```python
from build123d import *

# Parameters (mm, degrees)
ESQUISSE3_W              = 78
ESQUISSE3_H              = 56
BOSS_EXTRU_2_DEPTH       = 45
ESQUISSE4_R              = 34
ENL_V_MAT_EXTRU_1_DEPTH  = 30
ESQUISSE5_W              = 35.5
ESQUISSE5_H              = 35.5
ENL_V_MAT_EXTRU_2_DEPTH  = 15
ENL_V_MAT_EXTRU_5_DEPTH  = 10
ESQUISSE12_W             = 68
ESQUISSE12_H             = 18
ENL_V_MAT_EXTRU_6_DEPTH  = 30
ESQUISSE13_R             = 1.671466639
ENL_V_MAT_EXTRU_7_DEPTH  = 62.75
ESQUISSE15_R             = 1.5
ENL_V_MAT_EXTRU_8_DEPTH  = 62.75
ESQUISSE16_W             = 8
ESQUISSE16_H             = 8
ENL_V_MAT_EXTRU_9_DEPTH  = 4
ESQUISSE17_R             = 1.5
ENL_V_MAT_EXTRU_10_DEPTH = 41.5
ESQUISSE18_R             = 1.5
ENL_V_MAT_EXTRU_11_DEPTH = 41.5
ESQUISSE19_W             = 8
ESQUISSE19_H             = 8
ENL_V_MAT_EXTRU_12_DEPTH = 4
ENL_V_MAT_EXTRU_13_DEPTH = 46


with BuildPart() as part:
    # Esquisse3 → Boss.-Extru.2 (new body)
    with BuildSketch(Plane.XY):
        Rectangle(ESQUISSE3_W, ESQUISSE3_H)
    extrude(amount=BOSS_EXTRU_2_DEPTH)

    # Esquisse4 → Enlèv. mat.-Extru.1 (cut)
    with BuildSketch(Plane.XY.offset(45)):
        with Locations((0, -10)):
            Circle(ESQUISSE4_R)
    extrude(amount=-ENL_V_MAT_EXTRU_1_DEPTH, mode=Mode.SUBTRACT)

    # Esquisse5 → Enlèv. mat.-Extru.2 (cut)
    with BuildSketch(Plane(origin=(0, 0, 0), x_dir=(-1, 0, 0), z_dir=(0, 0, -1))):
        with Locations((0, -10.25)):
            Rectangle(ESQUISSE5_W, ESQUISSE5_H)
    extrude(amount=-ENL_V_MAT_EXTRU_2_DEPTH, mode=Mode.SUBTRACT)

    # Esquisse8 → Enlèv. mat.-Extru.5 (cut)
    with BuildSketch(Plane(origin=(0, 0, 0), x_dir=(-1, 0, 0), z_dir=(0, 0, -1))):
        Polygon((-22.75, -28), (-22.75, 12.5), (22.75, 12.5), (22.75, -28), (39, -28), (39, 28), (-39, 28), (-39, -28), align=None)
    extrude(amount=-ENL_V_MAT_EXTRU_5_DEPTH, mode=Mode.SUBTRACT)

    # Esquisse12 → Enlèv. mat.-Extru.6 (cut)
    with BuildSketch(Plane.XY.offset(45)):
        with Locations((0, -19)):
            Rectangle(ESQUISSE12_W, ESQUISSE12_H)
    extrude(amount=-ENL_V_MAT_EXTRU_6_DEPTH, mode=Mode.SUBTRACT)

    # Esquisse13 → Enlèv. mat.-Extru.7 (cut, through all)
    with BuildSketch(Plane.ZY.offset(22.75)):
        with Locations((5, -23)):
            Circle(ESQUISSE13_R)
    extrude(amount=-ENL_V_MAT_EXTRU_7_DEPTH, mode=Mode.SUBTRACT)

    # Esquisse15 → Enlèv. mat.-Extru.8 (cut, through all)
    with BuildSketch(Plane.ZY.offset(22.75)):
        with Locations((5, 2.5)):
            Circle(ESQUISSE15_R)
    extrude(amount=-ENL_V_MAT_EXTRU_8_DEPTH, mode=Mode.SUBTRACT)

    # Esquisse16 → Enlèv. mat.-Extru.9 (cut)
    with BuildSketch(Plane.XY.offset(15)):
        with Locations((-17.75, 7.5)):
            Rectangle(ESQUISSE16_W, ESQUISSE16_H)
    extrude(amount=-ENL_V_MAT_EXTRU_9_DEPTH, mode=Mode.SUBTRACT)

    # Esquisse17 → Enlèv. mat.-Extru.10 (cut, through all)
    with BuildSketch(Plane(origin=(0, 12.5, 0), x_dir=(1, 0, 0), z_dir=(0, 1, 0))):
        with Locations((-12.75, -5)):
            Circle(ESQUISSE17_R)
    extrude(amount=-ENL_V_MAT_EXTRU_10_DEPTH, mode=Mode.SUBTRACT)

    # Esquisse18 → Enlèv. mat.-Extru.11 (cut, through all)
    with BuildSketch(Plane(origin=(0, 12.5, 0), x_dir=(1, 0, 0), z_dir=(0, 1, 0))):
        with Locations((12.75, -5)):
            Circle(ESQUISSE18_R)
    extrude(amount=-ENL_V_MAT_EXTRU_11_DEPTH, mode=Mode.SUBTRACT)

    # Esquisse19 → Enlèv. mat.-Extru.12 (cut)
    with BuildSketch(Plane.XY.offset(15)):
        with Locations((17.75, 7.5)):
            Rectangle(ESQUISSE19_W, ESQUISSE19_H)
    extrude(amount=-ENL_V_MAT_EXTRU_12_DEPTH, mode=Mode.SUBTRACT)

    # Esquisse20 → Enlèv. mat.-Extru.13 (cut, through all)
    with BuildSketch(Plane.XY.offset(45)):
        Polygon((-39, 3), (-39, 28), (-14, 28), align=None)
    enl_v_mat_extru_13 = extrude(amount=-ENL_V_MAT_EXTRU_13_DEPTH, mode=Mode.SUBTRACT)

    # Symétrie1: Enlèv. mat.-Extru.13 across plane
    add(enl_v_mat_extru_13.mirror(Plane(origin=(0, 0, 0), x_dir=(0, 0, 1), z_dir=(1, 0, 0))), mode=Mode.SUBTRACT)


solid = part.part
```
Could you check a few things on this model? Use its own coordinates, in mm. A direction names the side the tool comes from. Give positions to 0.01 mm unless a question says otherwise; leave off trailing zeros. Order: outer loops, then holes, each group sorted by start corner. A loop starts at its lowest first (then second) coordinate and runs counter-clockwise, first axis right, second up.
Q1. I'm going to push flat-ended pins straight in: P1, Ø5, axis at x = -3.5, z = 6, coming from the +Y side; P2, Ø4.5, axis at y = 8, z = 13.5, coming from the +X side; P3, Ø10, axis at y = 12.5, z = 18, coming from the +X side; P4, Ø6, axis at x = -3.5, y = 6.5, coming from the -Z side. Where does each tip first touch, or does it pass through?
Q2. Suppose I cut it at D-D, the plane z = 12.5. Write out the boundary of the cut face in (x, y).
Q3. For faces 1 (the cylindrical face through (0.75, 23.99, 30.21)), 2 (the flat face through (0, 12.5, 5)), 3 (the flat face through (22.75, -8, 5)), which set-ups out of +Z, -Z, +X, -X, +Y, -Y let a thin tool reach every point of the face, with its end or its side?
Q4. If I drill on line 1 along X through (y, z) = (9.6, 5); line 2 along Y through (x, z) = (-20, 5); line 3 along Z through (x, y) = (-12.75, 10.5), over which ranges is the centre line in solid material (lowest first)?
Q5. Suppose I cut it at A-A, the plane y = -18. Write out the boundary of the cut face in (x, z).
Q6. Suppose I cut it at C-C, the plane x = -30. Write out the boundary of the cut face in (y, z).
Q7. Suppose I cut it at B-B, the plane z = 5. Count the separate pieces of the cut face and the enclosed holes in it, and give its area (3 significant figures).
Q8. We'd pull the mould along Y, two halves only. Please class faces 4 (the flat face through (19, 8, 11)), 5 (the flat face through (35, -28, 21)), 6 (the flat face through (-9, 23, 45)): +Y half, -Y half, draft (parallel to the pull), parting line (faces both ways), or undercut.
Solution:
1. P1: stops at y = 12.5
1. P2: stops at x = 36.25
1. P3: stops at x = 34.5
1. P4: stops at z = 0
2. outline: (-39, -28) - (-17.75, -28) - (-17.75, 3.5) - (-21.75, 3.5) - (-21.75, 11.5) - (-13.75, 11.5) - (-13.75, 7.5) - (13.75, 7.5) - (13.75, 11.5) - (21.75, 11.5) - (21.75, 3.5) - (17.75, 3.5) - (17.75, -28) - (39, -28) - (39, 3) - (14, 28) - (-14, 28) - (-39, 3) - close
3. face 1: +Z, -Y
3. face 2: -Z, +X, -X, +Y
3. face 3: -Z, +X, +Y, -Y
4. line 1: x = -22.75 to -14.25, -11.25 to 11.25, 14.25 to 22.75
4. line 2: y = -28 to -24.67, -21.33 to 1, 4 to 12.5
4. line 3: z = 0 to 3.5, 6.5 to 15
5. outline: (-39, 10) - (-22.75, 10) - (-22.75, 0) - (-17.75, 0) - (-17.75, 15) - (-34, 15) - (-34, 45) - (-39, 45) - close; (17.75, 0) - (22.75, 0) - (22.75, 10) - (39, 10) - (39, 45) - (34, 45) - (34, 15) - (17.75, 15) - close
6. outline: (-28, 10) - (12, 10) - (12, 45) - (6, 45) - (6, 15) - (-28, 15) - close
7. separate pieces: 7
7. enclosed holes: 0
7. area: 489 mm2
8. face 4: undercut
8. face 5: -Y half
8. face 6: draft
